Part model, mm, in its own coordinate system. A direction names the side the tool comes from. Round coordinates to 2 decimals unless told otherwise and drop trailing zeros. Loops run counter-clockwise (first coordinate to the right, second up) from the corner with the lowest first, then second, coordinate; pieces in that order, holes last.
from build123d import *

# Parameters (mm, degrees)
F0_W     = 1524
F0_H     = 2279.65
F1_DEPTH = 254
F2_W     = 1244.6
F2_H     = 406.4
F3_DEPTH = 25.4
F4_W     = 1244.6
F4_H     = 1333.5
F5_DEPTH = 50.8
F6_W     = 622.3
F6_H     = 774.7
F7_DEPTH = 12.7


with BuildPart() as f1:
    # F0 (on Front) → F1 (new body)
    with BuildSketch(Plane.XZ):
        with Locations((762, -1139.825)):
            Rectangle(F0_W, F0_H)
    extrude(amount=F1_DEPTH)

    # F2 (on face) → F3 (cut)
    with BuildSketch(Plane.XZ.offset(254)):
        with Locations((762, -381)):
            Rectangle(F2_W, F2_H)
    extrude(amount=-F3_DEPTH, mode=Mode.SUBTRACT)

    # F4 (on face) → F5 (cut)
    with BuildSketch(Plane.XZ.offset(254)):
        with Locations((762, -1333.5)):
            Rectangle(F4_W, F4_H)
    extrude(amount=-F5_DEPTH, mode=Mode.SUBTRACT)

    # F6 (on face) → F7 (join)
    with BuildSketch(Plane(origin=(0, 0, 0), x_dir=(-1, 0, 0), z_dir=(0, 1, 0))):
        with Locations((-755.65, -831.85)):
            Rectangle(F6_W, F6_H)
    extrude(amount=F7_DEPTH)


solid = f1.part
1) Wall check: line 1 along X through (y, z) = (-227.5, -1425.5); line 2 along Y through (x, z) = (1160.5, -1226); line 3 along Y through (x, z) = (1388, -1402.5). Give the ranges that are in metal, low to high.
Values:
line 1: x = 0 to 139.7, 1384.3 to 1524
line 2: y = -203.2 to 0
line 3: y = -254 to 0
2) Slice it at C-C, the plane x = 791. Give the cut face in (y, z).
Values:
outline: (-254, -2279.65) - (0, -2279.65) - (0, -1219.2) - (12.7, -1219.2) - (12.7, -444.5) - (0, -444.5) - (0, 0) - (-254, 0) - (-254, -177.8) - (-228.6, -177.8) - (-228.6, -584.2) - (-254, -584.2) - (-254, -666.75) - (-203.2, -666.75) - (-203.2, -2000.25) - (-254, -2000.25) - close
3) Slice it at D-D, the plane z = -1016. Give the cut face in (x, y).
Values:
outline: (0, -254) - (139.7, -254) - (139.7, -203.2) - (1384.3, -203.2) - (1384.3, -254) - (1524, -254) - (1524, 0) - (1066.8, 0) - (1066.8, 12.7) - (444.5, 12.7) - (444.5, 0) - (0, 0) - close
4) Slice it at B-B, the plane x = 412. Give the cut face in (y, z), then the cut area to 3 significant figures.
Values:
outline: (-254, -2279.65) - (0, -2279.65) - (0, 0) - (-254, 0) - (-254, -177.8) - (-228.6, -177.8) - (-228.6, -584.2) - (-254, -584.2) - (-254, -666.75) - (-203.2, -666.75) - (-203.2, -2000.25) - (-254, -2000.25) - close
area: 501,000 mm2
5) Slice it at A-A, the plane z = -1308. Give the cut face in (x, y), then the cut area to 3 significant figures.
Values:
outline: (0, -254) - (139.7, -254) - (139.7, -203.2) - (1384.3, -203.2) - (1384.3, -254) - (1524, -254) - (1524, 0) - (0, 0) - close
area: 324,000 mm2
6) Tool access for faces 1 (the face through (751, -125, -2279.65)), 2 (the face through (753, -228.6, -378)): list every direction of +Z, -Z, +X, -X, +Y, -Y with a clear straight run to the whole face (end or side of a thin tool).
Values:
face 1: -Z, +X, -X, +Y, -Y
face 2: -Y
7) Mould opens along X. For faces 3 (the face through (753, -203.2, -1324)), 4 (the face through (751, -254, -617)), 5 (the face through (139.7, -229, -1343)), 6 (the face through (0, -125, -1156)) say: released by +X, released by -X, zero draft, split by the parting line, or undercut.
Values:
face 3: undercut
face 4: zero draft
face 5: undercut
face 6: released by -X
8) Drop flat-ended pins along their axis: pin 1 Ø5 at (x, z) = (388, -654) entering from +Y; pin 2 Ø10 at (y, z) = (8.5, -739) entering from -X; pin 3 Ø6.5 at (x, y) = (650, 5.5) entering from -Z. Give the stop position or say it passes through.
Values:
pin 1: stops at y = 0
pin 2: stops at x = 444.5
pin 3: stops at z = -1219.2
